Solid Edge part; units mm, degrees
sketch "Sketch1" plane through (0, 0, 0) normal (0, 0, 1) x (1, 0, 0)
  line L0 (-13.8, -13.8) -> (13.8, -13.8)
  line L1 (13.8, -13.8) -> (13.8, 13.8)
  line L2 (13.8, 13.8) -> (-13.8, 13.8)
  line L3 (-13.8, 13.8) -> (-13.8, -13.8)
  dimension "D1" = 13.8
  dimension "D2" = 13.8
extrude "Protrusion1" add sketch "Sketch1" along normal blind 6
sketch "Sketch2" plane through (0, 0, 6) normal (0, 0, 1) x (1, 0, 0)
  line L0 (13.8, -11.3) -> (13.8, -13.8)
  line L1 (-11.3, -11.3) -> (13.8, -11.3)
  line L2 (-11.3, 11.3) -> (-11.3, -11.3)
  line L3 (11.3, 11.3) -> (-11.3, 11.3)
  line L4 (11.3, 3.7) -> (11.3, 11.3)
  line L5 (13.8, 3.7) -> (11.3, 3.7)
  line L6 (13.8, 13.8) -> (13.8, 3.7)
  line L7 (-13.8, 13.8) -> (13.8, 13.8)
  line L8 (-13.8, -13.8) -> (-13.8, 13.8)
  line L9 (13.8, -13.8) -> (-13.8, -13.8)
  dimension "D1" = 13.8
  dimension "D2" = 13.8
extrude "servo_holding" add sketch "Sketch2" along normal blind 11
sketch "Sketch3" plane through (1.25, 0, 5) normal (0, 0, 1) x (1, 0, 0)
  circle A0 centre (-3.1444, -0.8073) radius 1.25
extrude "Cutout1" cut sketch "Sketch3" against normal through all
sketch "Sketch4" plane through (0, 0, 17) normal (0, 0, 1) x (-1, 0, 0)
  line L0 (8.8, 13.8) -> (3.8, 13.8)
  line L1 (3.8, 13.8) -> (3.8, 11.3)
  line L2 (3.8, 11.3) -> (8.8, 11.3)
  line L3 (8.8, 11.3) -> (8.8, 13.8)
  dimension "D1" = 8.8
extrude "Cutout2" cut sketch "Sketch4" against normal up to vertex (11 mm away)
sketch "Sketch5" plane through (-13.8, 0, 8) normal (-1, 0, 0) x (0, 1, 0)
  circle A0 centre (-5.1, -4.2) radius 2.35
  circle A1 centre (-5.1, -4.2) radius 5
  dimension "D1" = 5.1
  dimension "D2" = 5.1
extrude "side_axis_mounting" add sketch "Sketch5" along normal blind 2.7
sketch "Sketch6" plane through (-16.5, -5.1, 11.2) normal (-1, 0, 0) x (0, 1, 0)
  circle A0 centre (0, -1) radius 2.35
extrude "Cutout3" cut sketch "Sketch6" against normal up to next
fillet "edges" radius 3 4 edges at (-13.8, -13.8, 8.5) (13.8, -13.8, 8.5) (13.8, 13.8, 8.5) (-13.8, 13.8, 8.5)
sketch "Sketch7" plane through (0, 0, 0) normal (0, 0, -1) x (0, 1, 0)
  line L0 (-2.5573, 6.6056) -> (0.9427, 6.6056)
  line L1 (0.9427, 6.6056) -> (0.9427, 1.2516)
  line L2 (0.9427, 1.2516) -> (11.8, 0.3945)
  line L3 (11.8, 0.3945) -> (11.8, -4.1833)
  line L4 (11.8, -4.1833) -> (0.9427, -5.0404)
  line L5 (0.9427, -10.3944) -> (0.9427, -5.0404)
  line L6 (-2.5573, -10.3944) -> (0.9427, -10.3944)
  line L7 (-2.5573, -10.3944) -> (-2.5573, -5.2944)
  line L8 (-11.8, -4.2795) -> (-2.5573, -5.2944)
  line L9 (-11.8, 0.4907) -> (-11.8, -4.2795)
  line L10 (-2.5573, 1.5056) -> (-11.8, 0.4907)
  line L11 (-2.5573, 6.6056) -> (-2.5573, 1.5056)
  dimension "D1" = 2.5573
  dimension "D2" = 2.5573
extrude "servo_cut" cut sketch "Sketch7" against normal blind 2.4
sketch "Sketch8" plane through (1.25, -1.25, 6) normal (0, 0, 1) x (-1, 0, 0)
  circle A0 centre (3.1444, -0.4427) radius 3
extrude "servo_screw_cut" cut sketch "Sketch8" against normal blind 5
sketch "Sketch9" plane through (-1.8944, 0, 2.4) normal (0, 0, -1) x (0.0787, 0.9969, 0)
  circle A0 centre (-0.8048, 0.0635) radius 3.4
extrude "Cutout4" cut sketch "Sketch9" against normal blind 0.4
sketch "Sketch10" plane through (0, 0, 0) normal (0, 0, -1) x (0, 1, 0)
  line L0 (-10.5067, 0.5392) -> (-13.1271, 0.2207)
  arc A0 (-13.1271, 0.2207) -> (11.4765, 0.42) centre (-0.8073, -1.8944) cw
  line L1 (8.815, 0.828) -> (11.4765, 0.42)
  arc A1 (-10.5067, 0.5392) -> (8.815, 0.828) centre (-0.8073, -1.8944) cw
  line L2 (-10.5056, -4.3325) -> (-13.1047, -4.1363)
  arc A2 (-13.1047, -4.1363) -> (11.4765, -4.2088) centre (-0.8073, -1.8944) ccw
  line L3 (8.8909, -4.3325) -> (11.4765, -4.2088)
  arc A3 (-10.5056, -4.3325) -> (8.8909, -4.3325) centre (-0.8073, -1.8944) ccw
extrude "Extrusionsausprägung_4" add sketch "Sketch10" along normal blind 9.6
chamfer "Fase_1" distance 1 angle 45 4 edges at (0.3799, -11.8169, -9.6) (0.624, 10.1457, -9.6) (-4.2706, 10.1837, -9.6) (-4.2344, -11.8051, -9.6)
sketch "Sketch11" plane through (0, -0.8073, 8.5) normal (0, -1, 0) x (-1, 0, 0)
  line L0 (14.3944, 8.5) -> (19.3944, 18.1)
  line L1 (19.3944, 18.1) -> (14.3944, 18.1)
  line L2 (14.3944, 18.1) -> (14.3944, 8.5)
  dimension "D1" = 19.3944
revolve "Rotationsausprägung_3" add sketch "Sketch11" angle 145 mid plane about axis through (-1.9507, -0.8073, -9.6) along (0, 0, 1)
sketch "Sketch12" plane through (0, 0, 17) normal (0, 0, 1) x (1, 0, 0)
  line L0 (10.3, 11.3) -> (11.3, 11.3)
  line L1 (11.3, 11.3) -> (11.3, 10.3)
  line L2 (12.0071, 11.0071) -> (11.3, 10.3)
  line L3 (11.0071, 12.0071) -> (12.0071, 11.0071)
  line L4 (10.3, 11.3) -> (11.0071, 12.0071)
  dimension "D1" = 10.3
  dimension "D2" = 10.3
extrude "Cutout5" cut sketch "Sketch12" against normal up to vertex (11 mm away)
mirror "Mirror1" about plane through (0, 0, 0) normal (1, 0, 0) of "Cutout5"
mirror "Mirror2" about plane through (0, 0, 0) normal (0, -1, 0) of "Cutout5", "Mirror1"
chamfer "Fase_2" distance 0.5 angle 45 1 edges at (-16.5, -7.45, 12.2)
sketch "Sketch13" plane through (0, -0.8073, 8.5) normal (0, -1, 0) x (-1, 0, 0)
  line L0 (-10.6056, 18.1) -> (-15.6056, 18.1)
  line L1 (-15.6056, 18.1) -> (-10.6056, 8.5)
  line L2 (-10.6056, 8.5) -> (-10.1056, 8.5)
  line L3 (-10.1056, 8.5) -> (-10.1056, 18.1)
  line L4 (-10.1056, 18.1) -> (-10.6056, 18.1)
  dimension "D1" = 10.6056
  dimension "D2" = 10.1056
revolve "Rotationsausprägung_5" add sketch "Sketch13" angle 145 mid plane about axis through (-2.2246, -0.8073, -9.6) along (0, 0, 1)
properties material "Nylon, allgemein"
The listing builds one solid part. Answer for the finished solid, in the listing's coordinates (mm). A direction names the side the tool comes from. Give positions to 0.01 mm unless a question says otherwise; leave off trailing zeros. Order: outer loops, then holes, each group sorted by start corner. A loop starts at its lowest first (then second) coordinate and runs counter-clockwise, first axis right, second up. Notation, with made-up numbers: (-3.75, -26.5) -> (44.25, -26.5) arc R18 ccw to (44.25, 0.5) -> close; hole circle Ø11 at (22, -4). An arc over 180 degrees is marked (long way). Answer as a JSON object with one key per item and string values. Group by question number.
Item 1: The part is cut by section A-A on z = 3.25. Write down the section's boundary in (x, y).
Item 2: Determine the mould class of faces 1 (the flat face through (-13.8, 3, 6)), 2 (the flat face through (8.3, -0.6, -9.6)), 3 (the flat face through (-11.3, 0, 11)), 4 (the cylindrical face through (-15.131, -5.751, 17.157)) for opening direction Z: pulls with the +Z half, pulls with the -Z half, needs draft (parallel to the pull), parting line crosses it, or undercut.
Item 3: A tool of negligible diameter and unlimited length cuts with its end or side. For faces 5 (the flat face through (0.38, -11.8, -4.24)), 6 (the flat face through (9, 6, 0)), 7 (the flat face through (-8.8, -13, 12)), 8 (the flat face through (11.5, 11.514, 11.577)), from which of +Z, -Z, +X, -X, +Y, -Y can it reach the whole face along a straight path? Write none if from no direction.
Item 4: The part is cut by section B-B on z = -5.25. Write down the section's boundary in (x, y) (1 decimal).
Item 5: Consider L1, parallel to Y at x = -14.3, z = 12.2; L2, parallel to Z at x = -14.1, y = -5.1; L3, parallel to Z at x = -14.4, y = -5.1. Determine where each line is inside the solid, lowest interval first. Write a range as from..to.
Item 6: Flat-ended cylindrical pins translate along their axes: pin 1 (2 mm diameter, centred on x = -13.5, y = 7.5, fed in from +Z); pin 2 (6 mm diameter, centred on y = -5.1, z = 12.2, fed in from -X); pin 3 (12 mm diameter, centred on x = 1.5, z = 12.5, fed in from -Y); pin 4 (3.5 mm diameter, centred on x = -1.89, y = -0.81, fed in from -Z). Find the tip coordinate at first contact, or state that the pin passes through.
Item 7: The part is cut by section C-C on z = 0.5. Write down the section's boundary in (x, y).
Item 8: The part is cut by section D-D on z = 12.2. Give the number of separate pieces and of enclosed holes in the cut face, and give its area (3 significant figures).
Result set:
{
 "1": {"outline": "(-13.8, -10.8) arc R3 ccw to (-10.8, -13.8) -> (10.8, -13.8) arc R3 ccw to (13.8, -10.8) -> (13.8, 10.8) arc R3 ccw to (10.8, 13.8) -> (-10.8, 13.8) arc R3 ccw to (-13.8, 10.8) -> close; hole circle Ø6 at (-1.89, -0.81)"},
 "2": {"face 1": "undercut", "face 2": "pulls with the -Z half", "face 3": "needs draft", "face 4": "undercut"},
 "3": {"face 5": "-Z", "face 6": "none", "face 7": "+Z, -Y", "face 8": "+Z"},
 "4": {"outline": "(-6.5, -15.3) -> (-5.7, -12.7) arc R12.5 ccw to (-4.1, -13.1) -> (-4.3, -10.5) arc R10 cw to (-4.3, 8.9) -> (-4.2, 11.5) arc R12.5 ccw to (-5.7, 11.1) -> (-6.5, 13.7) arc R15.2 ccw to start; (0.2, -13.1) arc R12.5 ccw to (1.6, -12.8) -> (2.5, -15.7) arc R15.6 ccw to (2.5, 14) -> (1.6, 11.2) arc R12.5 ccw to (0.4, 11.5) -> (0.8, 8.8) arc R10 cw to (0.5, -10.5) -> close"},
 "5": {"L1": "-10.1..-7.45, -2.75..-0.1", "L2": "-9.6..-0.85, 7.2..9.85, 14.55..17.2", "L3": "-9.6..-1.39, 7.2..9.85, 14.55..17.2"},
 "6": {"pin 1": "z = 17", "pin 2": "x = -16.5", "pin 3": "y = -13.8", "pin 4": "through"},
 "7": {"outline": "(-13.8, -10.8) arc R3 ccw to (-10.8, -13.8) -> (10.8, -13.8) arc R3 ccw to (13.8, -10.8) -> (13.8, 10.8) arc R3 ccw to (10.8, 13.8) -> (-10.8, 13.8) arc R3 ccw to (-13.8, 10.8) -> close; hole (-10.39, -2.56) -> (-5.29, -2.56) -> (-4.28, -11.8) -> (0.49, -11.8) -> (1.51, -2.56) -> (6.61, -2.56) -> (6.61, 0.94) -> (1.25, 0.94) -> (0.39, 11.8) -> (-4.18, 11.8) -> (-5.04, 0.94) -> (-10.39, 0.94) -> close"},
 "8": {"separate pieces": "3", "enclosed holes": "0", "area": "192 mm²"}
}
